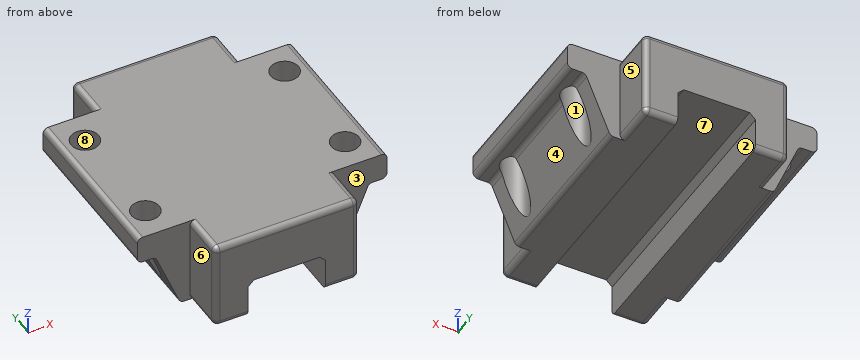
from build123d import *

# Parameters (mm, degrees)
F0_W          = 90
F0_H          = 32
F1_DEPTH      = 65.2
F3_DEPTH      = 25
F4_W          = 90
F4_H          = 65.2
F5_DEPTH      = 32.001
F6_DEPTH      = 62.5
F8_DEPTH      = 16.25
F8_DEPTH_BACK = 78.75
F9_R          = 2
F11_DEPTH     = 78.751
F12_R         = 5
F13_DEPTH     = 32.001


with BuildPart() as f1:
    # F0 (on Front) → F1 (new body)
    with BuildSketch(Plane.XZ):
        with Locations((-2.4301670492, -5.0586230417)):
            Rectangle(F0_W, F0_H)
    extrude(amount=F1_DEPTH)

    # F2 (on face) → F3 (join)
    with BuildSketch(Plane.XZ.offset(65.2)):
        with BuildLine():
            Line((40.5698329508, 10.9413769583), (-45.4301670492, 10.9413769583))
            ThreePointArc((-45.4301670492, 10.9413769583), (-46.8443806115, 10.3555905207), (-47.4301670492, 8.9413769583))
            Line((-47.4301670492, 8.9413769583), (-47.4301670492, 2.9413769583))
            ThreePointArc((-47.4301670492, 2.9413769583), (-46.8443806115, 1.5271633959), (-45.4301670492, 0.9413769583))
            Line((-45.4301670492, 0.9413769583), (-42.2728696535, 0.9413769583))
            ThreePointArc((-42.2728696535, 0.9413769583), (-41.1580897163, 0.6018785968), (-40.4217757411, -0.3013573503))
            Line((-40.4217757411, -0.3013573503), (-32.4385583572, -19.8158887331))
            ThreePointArc((-32.4385583572, -19.8158887331), (-31.7022443821, -20.7191246802), (-30.5874644448, -21.0586230417))
            Line((-30.5874644448, -21.0586230417), (25.7271303465, -21.0586230417))
            ThreePointArc((25.7271303465, -21.0586230417), (26.8419102837, -20.7191246802), (27.5782242589, -19.8158887331))
            Line((27.5782242589, -19.8158887331), (35.5614416428, -0.3013573503))
            ThreePointArc((35.5614416428, -0.3013573503), (36.2977556179, 0.6018785968), (37.4125355552, 0.9413769583))
            Line((37.4125355552, 0.9413769583), (40.5698329508, 0.9413769583))
            ThreePointArc((40.5698329508, 0.9413769583), (41.9840465132, 1.5271633959), (42.5698329508, 2.9413769583))
            Line((42.5698329508, 2.9413769583), (42.5698329508, 8.9413769583))
            ThreePointArc((42.5698329508, 8.9413769583), (41.9840465132, 10.3555905207), (40.5698329508, 10.9413769583))
        make_face()
    extrude(amount=F3_DEPTH)

    # F4 (on face) → F5 (cut, through all)
    with BuildSketch(Plane.XY.offset(10.9413769583)):
        with Locations((-2.4301670492, -32.6)):
            Rectangle(F4_W, F4_H)
    extrude(amount=-F5_DEPTH, mode=Mode.SUBTRACT)

    # F6 (add): a face of the model
    f6_faces = [f1.faces().sort_by_distance(p)[0] for p in [
        (-2.4301670492, -90.2, -3.7537517767),
    ]]
    extrude(f6_faces, amount=-F6_DEPTH)

    # F7 (on face) → F8 (join, two sides)
    with BuildSketch(Plane.XZ.offset(90.2)) as f8_sk:
        with BuildLine():
            Line((21.5698329508, 10.9413769583), (-26.4301670492, 10.9413769583))
            ThreePointArc((-26.4301670492, 10.9413769583), (-27.8443806115, 10.3555905207), (-28.4301670492, 8.9413769583))
            Line((-28.4301670492, 8.9413769583), (-28.4301670492, -19.0586230417))
            ThreePointArc((-28.4301670492, -19.0586230417), (-27.8443806115, -20.4728366041), (-26.4301670492, -21.0586230417))
            Line((-26.4301670492, -21.0586230417), (-16.4301670492, -21.0586230417))
            Line((-16.4301670492, -21.0586230417), (-16.4301670492, -9.1799433853))
            Line((-16.4301670492, -9.1799433853), (-14.3088467056, -7.0586230417))
            Line((-14.3088467056, -7.0586230417), (9.4485126073, -7.0586230417))
            Line((9.4485126073, -7.0586230417), (11.5698329508, -9.1799433853))
            Line((11.5698329508, -9.1799433853), (11.5698329508, -21.0586230417))
            Line((11.5698329508, -21.0586230417), (21.5698329508, -21.0586230417))
            ThreePointArc((21.5698329508, -21.0586230417), (22.9840465132, -20.4728366041), (23.5698329508, -19.0586230417))
            Line((23.5698329508, -19.0586230417), (23.5698329508, 8.9413769583))
            ThreePointArc((23.5698329508, 8.9413769583), (22.9840465132, 10.3555905207), (21.5698329508, 10.9413769583))
        make_face()
    extrude(amount=F8_DEPTH)
    extrude(f8_sk.sketch, amount=-F8_DEPTH_BACK)

    # F9
    f9_edges = [f1.edges().sort_by_distance(p)[0] for p in [
        (-28.430167, -106.45, -5.058623),
        (-2.430167, -11.45, 10.941377),
    ]]
    fillet(f9_edges, radius=F9_R)

    # F10 (on face) → F11 (cut, through all)
    with BuildSketch(Plane.XZ.offset(90.2)):
        Polygon((-16.4301670492, -9.1799433853), (-16.4301670492, -21.0586230417), (11.5698329508, -21.0586230417), (11.5698329508, -9.1799433853), (9.4485126073, -7.0586230417), (-14.3088467056, -7.0586230417), align=None)
    extrude(amount=-F11_DEPTH, mode=Mode.SUBTRACT)

    # F12 (on face) → F13 (cut, through all)
    with BuildSketch(Plane.XY.offset(10.9413769583)):
        with Locations((-38.4301670492, -38.95)):
            Circle(F12_R)
        with Locations((-38.4301670492, -78.95)):
            Circle(F12_R)
        with Locations((33.5698329508, -78.95)):
            Circle(F12_R)
        with Locations((33.5698329508, -38.95)):
            Circle(F12_R)
    extrude(amount=-F13_DEPTH, mode=Mode.SUBTRACT)


solid = f1.part
The listing builds one solid part. Answer for the finished solid, in the listing's coordinates (mm). Face numbers are marked on the shaded views. A direction names the side the tool comes from. Give positions to 0.01 mm unless a question says otherwise; leave off trailing zeros. Write each loop counter-clockwise with the first axis right and the second up, starting at its lowest first coordinate (ties: lowest second). Pieces come first, ordered by that corner, then holes.
1) Section C-C (y = -57.5) is taken. Write down the section's boundary in (x, z).
2) Section A-A (z = 5) is taken. Write down the section's boundary in (x, y).
3) Find the intervals of material crossed by L1, parallel to X at y = -78.95, z = 4; L2, parallel to X at y = -26, z = -11.5; L3, parallel to X at y = -78.95, z = -0.25, in increasing order.
4) Section D-D (z = -11.5) is taken. Write down the section's boundary in (x, y).
5) Section B-B (y = -38.95) is taken. Write down the section's boundary in (x, z).
6) A tool of negligible diameter and unlimited length cuts with its end or side. For the marked faces 5, 6, 7 and 8, from which of +Z, -Z, +X, -X, +Y, -Y can it reach the whole face along a straight path? Write none if from no direction.
7) Given P1, Ø1.5, axis at y = -62, z = -11, coming from the +X side; P2, Ø4, axis at y = -78.5, z = -5.5, coming from the +X side; P3, Ø7, axis at y = -98.5, z = -4.5, coming from the -X side, each flat-ended and moving along its own axis, determine where each tip first touches the part or whether it passes through.
8) For a pull along X with two mould halves and no side action, classify the marked faces 1, 2, 3 and 4 as pulls with the +X half, pulls with the -X half, needs draft (parallel to the pull), parting line crosses it, or undercut.
Response:
1. outline: (-47.43, 2.94) arc R2 ccw to (-45.43, 0.94) - (-42.27, 0.94) arc R2 cw to (-40.42, -0.3) - (-32.44, -19.82) arc R2 ccw to (-30.59, -21.06) - (-16.43, -21.06) - (-16.43, -9.18) - (-14.31, -7.06) - (9.45, -7.06) - (11.57, -9.18) - (11.57, -21.06) - (25.73, -21.06) arc R2 ccw to (27.58, -19.82) - (35.56, -0.3) arc R2 cw to (37.41, 0.94) - (40.57, 0.94) arc R2 ccw to (42.57, 2.94) - (42.57, 8.94) arc R2 ccw to (40.57, 10.94) - (-45.43, 10.94) arc R2 ccw to (-47.43, 8.94) - close
2. outline: (-47.43, -90.2) - (-28.43, -90.2) - (-28.43, -104.45) arc R2 ccw to (-26.43, -106.45) - (21.57, -106.45) arc R2 ccw to (23.57, -104.45) - (23.57, -90.2) - (42.57, -90.2) - (42.57, -27.7) - (23.57, -27.7) - (23.57, -13.45) arc R2 ccw to (21.57, -11.45) - (-26.43, -11.45) arc R2 ccw to (-28.43, -13.45) - (-28.43, -27.7) - (-47.43, -27.7) - close; hole circle Ø10 at (-38.43, -78.95); hole circle Ø10 at (-38.43, -38.95); hole circle Ø10 at (33.57, -78.95); hole circle Ø10 at (33.57, -38.95)
3. L1: x = -47.43 to -43.43, -33.43 to 28.57, 38.57 to 42.57
3. L2: x = -28.43 to -16.43, 11.57 to 23.57
3. L3: x = -33.43 to 28.57
4. outline: (-35.84, -90.2) - (-28.43, -90.2) - (-28.43, -104.45) arc R2 ccw to (-26.43, -106.45) - (-16.43, -106.45) - (-16.43, -11.45) - (-26.43, -11.45) arc R2 ccw to (-28.43, -13.45) - (-28.43, -27.7) - (-35.84, -27.7) - (-35.84, -34.67) arc R5 cw to (-35.84, -43.23) - (-35.84, -74.67) arc R5 cw to (-35.84, -83.23) - close; (11.57, -106.45) - (21.57, -106.45) arc R2 ccw to (23.57, -104.45) - (23.57, -90.2) - (30.98, -90.2) - (30.98, -83.23) arc R5 cw to (30.98, -74.67) - (30.98, -43.23) arc R5 cw to (30.98, -34.67) - (30.98, -27.7) - (23.57, -27.7) - (23.57, -13.45) arc R2 ccw to (21.57, -11.45) - (11.57, -11.45) - close
5. outline: (-47.43, 2.94) arc R2 ccw to (-45.43, 0.94) - (-43.43, 0.94) - (-43.43, 10.94) - (-45.43, 10.94) arc R2 ccw to (-47.43, 8.94) - close; (-33.43, -17.39) - (-32.44, -19.82) arc R2 ccw to (-30.59, -21.06) - (-16.43, -21.06) - (-16.43, -9.18) - (-14.31, -7.06) - (9.45, -7.06) - (11.57, -9.18) - (11.57, -21.06) - (25.73, -21.06) arc R2 ccw to (27.58, -19.82) - (28.57, -17.39) - (28.57, 10.94) - (-33.43, 10.94) - close; (38.57, 0.94) - (40.57, 0.94) arc R2 ccw to (42.57, 2.94) - (42.57, 8.94) arc R2 ccw to (40.57, 10.94) - (38.57, 10.94) - close
6. face 5: +Z, -Z, +X, +Y
6. face 6: +Z, -Z, -X, -Y
6. face 7: -Z, +Y, -Y
6. face 8: +Z, -Z
7. P1: stops at x = 31.49
7. P2: stops at x = 29.21
7. P3: stops at x = -28.43
8. face 1: undercut
8. face 2: undercut
8. face 3: needs draft
8. face 4: pulls with the +X half
